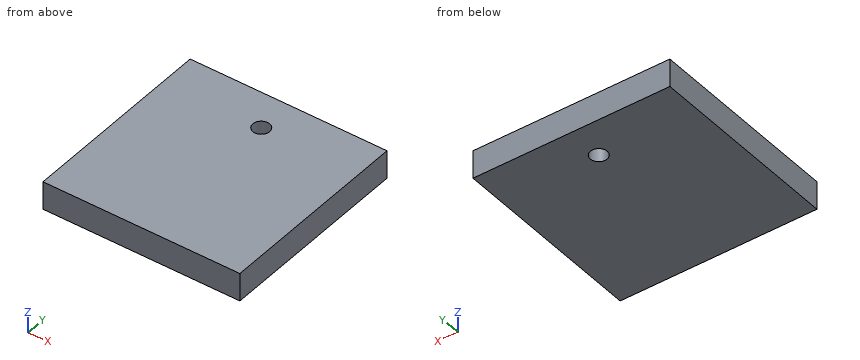
```python
from build123d import *

# Parameters (mm, degrees)
SKETCH2_W               = 35
SKETCH2_H               = 35
BOSS_EXTRUDE1_DEPTH     = 5
CUT_EXTRUDE1_DEPTH      = 26.248762346
CUT_EXTRUDE1_DEPTH_BACK = 26.248762346
SKETCH3_R               = 1.5


with BuildPart() as part:
    # Sketch2 → Boss-Extrude1 (new body)
    with BuildSketch(Plane.XY):
        Rectangle(SKETCH2_W, SKETCH2_H)
    extrude(amount=BOSS_EXTRUDE1_DEPTH)

    # Sketch3 → Cut-Extrude1 (cut, two sides: drawn at the far end of the back side and taken through both)
    with BuildSketch(Plane.XY.offset(5).offset(-CUT_EXTRUDE1_DEPTH_BACK)):
        with Locations((0, 11)):
            Circle(SKETCH3_R)
    extrude(amount=CUT_EXTRUDE1_DEPTH + CUT_EXTRUDE1_DEPTH_BACK, mode=Mode.SUBTRACT)


solid = part.part
```
The listing builds one solid part. Answer for the finished solid, in the listing's coordinates (mm). Give positions to 0.01 mm unless a question says otherwise; leave off trailing zeros. Order: outer loops, then holes, each group sorted by start corner. A loop starts at its lowest first (then second) coordinate and runs counter-clockwise, first axis right, second up. Notation, with made-up numbers: M 35.5,49.5 L 85.5,49.5 A16 cw 85.5,80.5 Z; hole C -4.75,19 d11. An arc over 180 degrees is marked long. Put each result on its own line as item: value. Start each with the question number.
Item 1: The part is cut by section B-B, the plane y = 11. Determine the outline of the cut face in (x, z), and give its area (3 significant figures).
Item 2: A flat-ended cylindrical pin translates along its axis: P1, Ø2.5, axis at x = 0, y = 11, coming from the +Z side. Find the tip coordinate at first contact, or state that the pin passes through.
Item 3: The part is cut by section A-A, the plane x = 0. Determine the outline of the cut face in (y, z).
Item 4: Find the intervals of material crossed by line 1 along Y through (x, z) = (0, 3.5); line 2 along X through (y, z) = (11, 2); line 3 along Y through (x, z) = (0.5, 0.85), in increasing order.
Answer key:
1. outline: M -17.5,0 L -1.5,0 L -1.5,5 L -17.5,5 Z; M 1.5,0 L 17.5,0 L 17.5,5 L 1.5,5 Z
1. area: 160 mm²
2. P1: passes through
3. outline: M -17.5,0 L 9.5,0 L 9.5,5 L -17.5,5 Z; M 12.5,0 L 17.5,0 L 17.5,5 L 12.5,5 Z
4. line 1: y = -17.5 to 9.5, 12.5 to 17.5
4. line 2: x = -17.5 to -1.5, 1.5 to 17.5
4. line 3: y = -17.5 to 9.59, 12.41 to 17.5
